Autodesk Inventor part; units mm, degrees
ref_plane "YZ Plane" through (0, 0, 0) normal (1, 0, 0) x (0, 1, 0)
ref_plane "XZ Plane" through (0, 0, 0) normal (0, 1, 0) x (-1, 0, 0)
ref_plane "XY Plane" through (0, 0, 0) normal (0, 0, 1) x (1, 0, 0)
sketch "Sketch1" plane through (0, 0, 0) normal (0, 1, 0) x (-1, 0, 0)
  line L0 (34.75, 22.5) -> (34.75, -22.5)
  line L1 (-34.75, 22.5) -> (-34.75, -22.5)
  line L2 (34.75, -22.5) -> (26, -22.5)
  line L3 (-34.75, -22.5) -> (-26, -22.5)
  line L4 (34.75, 22.5) -> (26, 22.5)
  line L5 (-34.75, 22.5) -> (-26, 22.5)
  line L6 (-26, -22.5) -> (-26, -55)
  line L7 (26, -22.5) -> (26, -55)
  line L8 (26, 22.5) -> (26, 55)
  line L9 (-26, 22.5) -> (-26, 55)
  line L10 (26, 55) -> (-26, 55)
  line L11 (26, -55) -> (-26, -55)
  point P0 (0, 0)
  dimension "d0" = 45
  dimension "d1" = 34.75
  dimension "d2" = 22.5
  dimension "d3" = 45
  dimension "d4" = 34.75
  dimension "d5" = 22.5
  dimension "d6" = 8.75
  dimension "d7" = 8.75
  dimension "d8" = 8.75
  dimension "d9" = 8.75
  dimension "d10" = 32.5
  dimension "d11" = 32.5
  dimension "d12" = 32.5
  dimension "d13" = 32.5
extrude "Extrusion1" add sketch "Sketch1" along normal blind 2
sketch "Sketch2" plane through (34.75, 0, 22.5) normal (1, 0, 0) x (0, 0, -1)
  line L0 (45, 2) -> (77.5, 2)
  line L1 (45, 2) -> (0, 2)
  line L2 (45, 2) -> (0, 2)
  line L3 (0, 2) -> (0, -6)
  line L4 (1, -7) -> (44, -7)
  line L5 (45, -6) -> (45, 2)
  line L6 (7.5, -4) -> (37.5, -4) construction
  circle A0 centre (7.5, -4) radius 1.25
  circle A1 centre (37.5, -4) radius 1.25
  arc A2 (0, -6) -> (1, -7) centre (1, -6) ccw
  arc A3 (44, -7) -> (45, -6) centre (44, -6) ccw
  point P0 (22.5, 0)
  point P1 (0, -7)
  point P2 (45, -7)
  dimension "d16" = 9
  dimension "d17" = 45
  dimension "d18" = 30
  dimension "d19" = 3
  dimension "d20" = 7.5
  dimension "d21" = 2.5
  dimension "d22" = 2.5
  dimension "d23" = 1
  dimension "d24" = 1
extrude "Extrusion2" add sketch "Sketch2" against normal blind 2
sketch "Sketch3" plane through (-34.75, 0, -22.5) normal (-1, 0, 0) x (0, 0, 1)
  line L0 (-32.5, 2) -> (0, 2)
  line L1 (0, 2) -> (45, 2)
  line L2 (45, 2) -> (45, -6)
  line L3 (44, -7) -> (1, -7)
  line L4 (0, -6) -> (0, 2)
  circle A0 centre (37.5, -4) radius 1.25
  circle A1 centre (37.5, -4) radius 1.25
  circle A2 centre (7.5, -4) radius 1.25
  circle A3 centre (7.5, -4) radius 1.25
  arc A4 (0, -6) -> (1, -7) centre (1, -6) ccw
  arc A5 (44, -7) -> (45, -6) centre (44, -6) ccw
  point P0 (22.5, 0)
  point P1 (45, -7)
  point P2 (0, -7)
  dimension "d27" = 45
  dimension "d28" = 9
  dimension "d29" = 1
extrude "Extrusion3" add sketch "Sketch3" against normal blind 2
sketch "Sketch4" plane through (26, 0, -22.5) normal (1, 0, 0) x (0, 0, -1)
  line L0 (32.5, 2) -> (0, 2)
  line L1 (7.5, 2) -> (7.5, -5)
  line L2 (8.5, -6) -> (31.5, -6)
  line L3 (32.5, -5) -> (32.5, 2)
  line L4 (12.5, -3) -> (27.5, -3)
  line L5 (11.5, -2) -> (11.5, 2)
  line L6 (28.5, -2) -> (28.5, 2)
  line L7 (32.5, 2) -> (28.5, 2)
  line L8 (11.5, 2) -> (7.5, 2)
  arc A0 (7.5, -5) -> (8.5, -6) centre (8.5, -5) ccw
  arc A1 (11.5, -2) -> (12.5, -3) centre (12.5, -2) ccw
  arc A2 (27.5, -3) -> (28.5, -2) centre (27.5, -2) ccw
  arc A3 (31.5, -6) -> (32.5, -5) centre (31.5, -5) ccw
  point P0 (-22.5, 0)
  point P1 (7.5, -6)
  point P2 (32.5, -6)
  point P3 (11.5, -3)
  point P4 (28.5, -3)
  dimension "d32" = 25
  dimension "d33" = 8
  dimension "d34" = 17
  dimension "d35" = 4
  dimension "d36" = 3
  dimension "d37" = 8
  dimension "d38" = 1
extrude "Extrusion4" add sketch "Sketch4" against normal blind 2 contours L3 A3 L2 A0 L1 L0 L5 A1 L4 A2 L6
sketch "Sketch5" plane through (26, 0, 55) normal (1, 0, 0) x (0, 0, -1)
  line L0 (0, 2) -> (32.5, 2)
  line L1 (25, 2) -> (25, -5)
  line L2 (24, -6) -> (1, -6)
  line L3 (0, -5) -> (0, 2)
  line L4 (5, -3) -> (20, -3)
  line L5 (4, -2) -> (4, 2)
  line L6 (21, -2) -> (21, 2)
  line L7 (0, 2) -> (4, 2)
  line L8 (21, 2) -> (25, 2)
  arc A0 (0, -5) -> (1, -6) centre (1, -5) ccw
  arc A1 (24, -6) -> (25, -5) centre (24, -5) ccw
  arc A2 (4, -2) -> (5, -3) centre (5, -2) ccw
  arc A3 (20, -3) -> (21, -2) centre (20, -2) ccw
  point P0 (55, 0)
  point P1 (25, -6)
  point P2 (0, -6)
  point P3 (4, -3)
  point P4 (21, -3)
  dimension "d41" = 25
  dimension "d42" = 8
  dimension "d43" = 17
  dimension "d44" = 5
  dimension "d45" = 4
  dimension "d46" = 8
  dimension "d47" = 1
  dimension "d65" = 1
extrude "Extrusion5" add sketch "Sketch5" against normal blind 2 contours L0 L5 A2 L4 A3 L6 L1 A1 L2 A0 L3
sketch "Sketch6" plane through (-26, 0, 22.5) normal (-1, 0, 0) x (0, 0, 1)
  line L0 (32.5, 0) -> (32.5, 2)
  line L1 (32.5, 2) -> (7.5, 2) construction
  line L2 (7.5, 2) -> (7.5, -5)
  line L3 (8.5, -6) -> (31.5, -6)
  line L4 (32.5, -5) -> (32.5, 2)
  line L5 (27.5, -3) -> (12.5, -3)
  line L6 (28.5, -2) -> (28.5, 2)
  line L7 (0, 2) -> (32.5, 2)
  line L8 (11.5, -2) -> (11.5, 2)
  line L9 (32.5, 2) -> (28.5, 2)
  line L10 (11.5, 2) -> (7.5, 2)
  arc A0 (31.5, -6) -> (32.5, -5) centre (31.5, -5) ccw
  arc A1 (7.5, -5) -> (8.5, -6) centre (8.5, -5) ccw
  arc A2 (11.5, -2) -> (12.5, -3) centre (12.5, -2) ccw
  arc A3 (27.5, -3) -> (28.5, -2) centre (27.5, -2) ccw
  line L11 (-77.5, 2) -> (-45, 2) construction
  line L12 (-77.5, 2) -> (-52.5, 2) construction
  line L13 (-52.5, 2) -> (-52.5, -5)
  line L14 (-53.5, -6) -> (-76.5, -6)
  line L15 (-77.5, -5) -> (-77.5, 2)
  line L16 (-57.5, -3) -> (-72.5, -3)
  line L17 (-56.5, -2) -> (-56.5, 2)
  line L18 (-73.5, -2) -> (-73.5, 2)
  line L19 (-52.5, 2) -> (-56.5, 2)
  line L20 (-73.5, 2) -> (-77.5, 2)
  arc A4 (-53.5, -6) -> (-52.5, -5) centre (-53.5, -5) ccw
  arc A5 (-57.5, -3) -> (-56.5, -2) centre (-57.5, -2) ccw
  arc A6 (-73.5, -2) -> (-72.5, -3) centre (-72.5, -2) ccw
  arc A7 (-77.5, -5) -> (-76.5, -6) centre (-76.5, -5) ccw
  point P0 (-22.5, 0)
  point P1 (7.5, -6)
  point P2 (32.5, -6)
  point P3 (28.5, -3)
  point P4 (11.5, -3)
  point P5 (-52.5, -6)
  point P6 (-77.5, -6)
  point P7 (-56.5, -3)
  point P8 (-73.5, -3)
  dimension "d50" = 25
  dimension "d51" = 8
  dimension "d52" = 17
  dimension "d53" = 4
  dimension "d54" = 3
  dimension "d55" = 1
  dimension "d56" = 1
  dimension "d57" = 1
  dimension "d58" = 1
  dimension "d59" = 25
  dimension "d60" = 8
  dimension "d61" = 17
  dimension "d62" = 4
  dimension "d63" = 3
  dimension "d64" = 1
extrude "Extrusion6" add sketch "Sketch6" against normal blind 2 contours L4 A0 L3 A1 L2 L7 L8 A2 L5 A3 L6 L0 | L13 A4 L14 A7 L15 L20 L18 A6 L16 A5 L17 L19
properties part number "RCT-H112_stick_battery_plate"
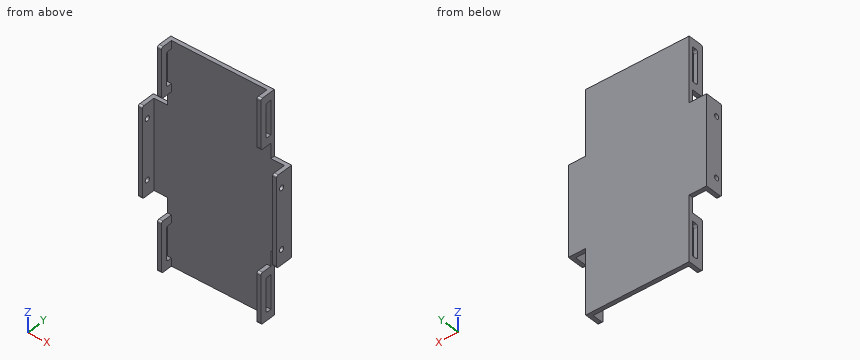
Here's how the part is built. I have some questions about the finished solid (model axes, mm). Round coordinates to 2 decimals unless told otherwise and drop trailing zeros. Order: outer loops, then holes, each group sorted by start corner. A loop starts at its lowest first (then second) coordinate and runs counter-clockwise, first axis right, second up. Notation, with made-up numbers: M -33,38.5 L -28,38.5 A13 ccw -28,61.5 Z; hole C -22.5,18.5 d2. An arc over 180 degrees is marked long. Answer as CSV lines item,"result".
Item 1: Imagine slicing it at B-B on z = -15. List the corners of the cut face in (x, y) for me, and give its area (3 significant figures).
From the geometry:
outline,"M -34.75,-7 L -32.75,-7 L -32.75,-5.25 L -34.75,-5.25 Z; M -34.75,-2.75 L -32.75,-2.75 L -32.75,0 L 32.75,0 L 32.75,-2.75 L 34.75,-2.75 L 34.75,2 L -34.75,2 Z; M 32.75,-7 L 34.75,-7 L 34.75,-5.25 L 32.75,-5.25 Z"
area,"157 mm2"
Item 2: Please list where these lines run through material, in increasing order: L1, parallel to X at y = -0.25, z = -4.5; L2, parallel to Y at x = -34.25, z = 15; L3, parallel to X at y = -5.5, z = -39. Write a range as [from, to].
From the geometry:
L1,"[-34.75, -32.75], [32.75, 34.75]"
L2,"[-7, -5.25], [-2.75, 2]"
L3,"[-26, -24], [24, 26]"
Item 3: Imagine slicing it at A-A on z = 37. List the corners of the cut face in (x, y) for me.
From the geometry:
outline,"M -26,-6 L -24,-6 L -24,-3 L -26,-3 Z; M -26,0 L 26,0 L 26,2 L -26,2 Z; M 24,-6 L 26,-6 L 26,-3 L 24,-3 Z"
Item 4: For pin 1 (8 mm diameter, centred on x = -4.5, z = -7.5, fed in from -Y); pin 2 (5 mm diameter, centred on y = -3.5, z = 44, fed in from -X); pin 3 (2.5 mm diameter, centred on x = 32.5, y = -3.5, fed in from +Z), each with a flat end and sliding along its axis, tell me the tip position at first contact or that it passes through.
From the geometry:
pin 1,"y = 0"
pin 2,"x = -26"
pin 3,"z = 22.5"
Item 5: Imagine slicing it at C-C on x = -6.5. List the corners of the cut face in (y, z) for me, and give its area (3 significant figures).
From the geometry:
outline,"M 0,-55 L 2,-55 L 2,55 L 0,55 Z"
area,"220 mm2"
